```python
from build123d import *

# Parameters (mm, degrees)
ESQUISSE1_R             = 5
BOSS_EXTRU_1_DEPTH      = 5
ESQUISSE6_R             = 35
ESQUISSE6_R_2           = 30
BOSS_EXTRU_6_DEPTH      = 5
BOSS_EXTRU_9_DEPTH      = 30
CONG_3_R                = 5
ESQUISSE10_R            = 2.6
ENL_V_MAT_EXTRU_1_DEPTH = 87.782774789


with BuildPart() as part:
    # Esquisse1 → Boss.-Extru.1 (new body)
    with BuildSketch(Plane.XY):
        with BuildLine():
            Line((-45.620718977, 15), (-70, 15))
            Line((-70, 15), (-70, -15))
            Line((-70, -15), (-45.620718977, -15))
            ThreePointArc((-45.620718977, -15), (-36.774201608, -17.062911874), (-29.752642811, -22.826086957))
            ThreePointArc((-29.752642811, -22.826086957), (37.5, 0), (-29.752642811, 22.826086957))
            ThreePointArc((-29.752642811, 22.826086957), (-36.774201608, 17.062911874), (-45.620718977, 15))
        make_face()
        Circle(ESQUISSE1_R, mode=Mode.SUBTRACT)
    extrude(amount=BOSS_EXTRU_1_DEPTH)

    # Esquisse6 → Boss.-Extru.6 (add)
    with BuildSketch(Plane.XY.offset(5)):
        Circle(ESQUISSE6_R)
        Circle(ESQUISSE6_R_2, mode=Mode.SUBTRACT)
    extrude(amount=BOSS_EXTRU_6_DEPTH)

    # Esquisse8 → Boss.-Extru.9 (add)
    with BuildSketch(Plane.XY.offset(5)):
        with BuildLine():
            Line((-70, -15), (-70, 15))
            Line((-70, 15), (-43.874821937, 15))
            ThreePointArc((-43.874821937, 15), (-39.966142137, 13.118047822), (-38.999841722, 8.888888889))
            ThreePointArc((-38.999841722, 8.888888889), (-40, 0), (-38.999841722, -8.888888889))
            ThreePointArc((-38.999841722, -8.888888889), (-39.966142137, -13.118047822), (-43.874821937, -15))
            Line((-43.874821937, -15), (-70, -15))
        make_face()
    extrude(amount=BOSS_EXTRU_9_DEPTH)

    # Congé3
    cong_3_edges = [part.edges().sort_by_distance(p)[0] for p in [
        (37.5, 0, 0),
        (-57.810359489, 15, 0),
        (-57.810359489, -15, 0),
        (-36.774201608, -17.062911874, 0),
        (-36.774201608, 17.062911874, 0),
    ]]
    fillet(cong_3_edges, radius=CONG_3_R - 0.0001)  # a hair under: the kernel refuses the full size

    # Esquisse10 → Enlèv. mat.-Extru.1 (cut, through all)
    with BuildSketch(Plane(origin=(0, 0, 0), x_dir=(-1, 0, 0), z_dir=(0, 0, -1))):
        with Locations((-15.40723238, 7.18451045)):
            Circle(ESQUISSE10_R)
        with Locations((7.18451045, 15.40723238)):
            Circle(ESQUISSE10_R)
        with Locations((15.40723238, -7.18451045)):
            Circle(ESQUISSE10_R)
        with Locations((-7.18451045, -15.40723238)):
            Circle(ESQUISSE10_R)
    extrude(amount=-ENL_V_MAT_EXTRU_1_DEPTH, mode=Mode.SUBTRACT)


solid = part.part
```
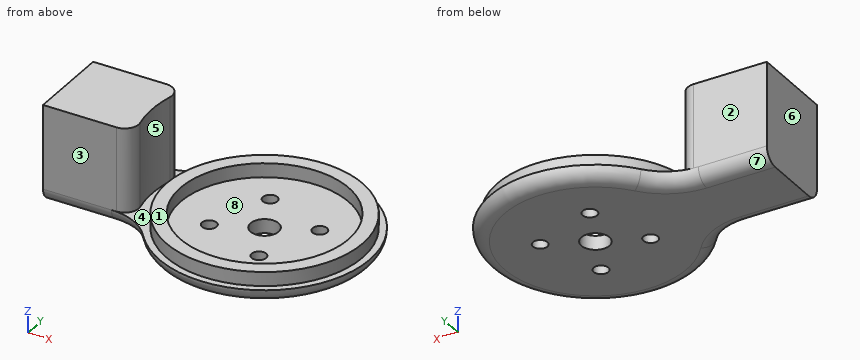
Design review of the part built by this model. Coordinates are the model's own, in mm. Face numbers are marked on the shaded views. A direction names the side the tool comes from. Give positions to 0.01 mm unless a question says otherwise; leave off trailing zeros. Write each loop counter-clockwise with the first axis right and the second up, starting at its lowest first coordinate (ties: lowest second). Pieces come first, ordered by that corner, then holes. Notation, with made-up numbers: (62, -30) -> (92, -30) arc R21 ccw to (92, -26) -> close; hole circle Ø10 at (69, 26). An arc over 180 degrees is marked (long way). Answer in a Markdown table with one row per item.
(1) Consider section D-D (z = 19). State the section outline as (x, y) points, then the cut area to 3 significant figures.
Results:
| item | result |
|---|---|
| outline | (-70, -15) -> (-43.87, -15) arc R5 ccw to (-39, -8.89) arc R40 cw to (-39, 8.89) arc R5 ccw to (-43.87, 15) -> (-70, 15) -> close |
| area | 909 mm2 |
(2) To check wall thickness, follow probe 1 along Z at (x, y) = (-21.5, -17.5); probe 2 along Z at (x, y) = (22, -24.5); probe 3 along Y at (x, z) = (-57.5, 18.5). State the ranges of each line that lie inside material, in increasing order.
Results:
| item | result |
|---|---|
| probe 1 | 0 to 5 |
| probe 2 | 0.02 to 10 |
| probe 3 | -15 to 15 |
(3) Consider section C-C (x = -63.5). State the section outline as (y, z) points.
Results:
| item | result |
|---|---|
| outline | (-15, 5) arc R5 ccw to (-10, 0) -> (10, 0) arc R5 ccw to (15, 5) -> (15, 35) -> (-15, 35) -> close |
(4) For the marked faces 1, 2, 3 and 4, list the 3-axis set-ups (+Z, -Z, +X, -X, +Y, -Y) from which the entire face can be reached by the end or side of a thin tool; tool diameter is ignored.
Results:
| item | result |
|---|---|
| face 1 | +Z, +X, +Y, -Y |
| face 2 | +Z, -Z, -X, +Y |
| face 3 | +Z, -Z, -X, -Y |
| face 4 | +Z |
(5) Clearance check with flat-ended pins moving along their axes: pin 1 (10 mm diameter, centred on x = -1, y = 13.5, fed in from +Z); pin 2 (21 mm diameter, centred on x = -58.5, z = 23, fed in from +Y); pin 3 (5 mm diameter, centred on x = -11, y = -26.5, fed in from +Z). State where each tip first meets the part, or that it passes through.
Results:
| item | result |
|---|---|
| pin 1 | z = 5 |
| pin 2 | y = 15 |
| pin 3 | z = 10 |
(6) Consider section A-A (z = 8.5). State the section outline as (x, y) points.
Results:
| item | result |
|---|---|
| outline | (-70, -15) -> (-43.87, -15) arc R5 ccw to (-39, -8.89) arc R40 cw to (-39, 8.89) arc R5 ccw to (-43.87, 15) -> (-70, 15) -> close; circle Ø70 at (0, 0); hole circle Ø60 at (0, 0) |
(7) Mouldability with a two-part tool opening along Y and no side actions: class the marked faces 5, 6, 7 and 8 as +Y half, -Y half, draft (parallel to the pull), parting line (faces both ways), or undercut.
Results:
| item | result |
|---|---|
| face 5 | undercut |
| face 6 | draft |
| face 7 | +Y half |
| face 8 | undercut |
